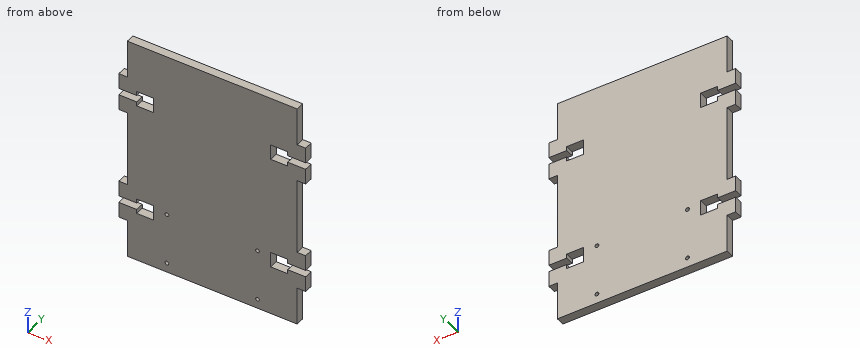
from build123d import *

# Parameters (mm, degrees)
SKETCH1_W           = 90
SKETCH1_H           = 20
SKETCH1_W_2         = 4.5
SKETCH1_H_2         = 8.2
SKETCH1_W_3         = 62
SKETCH1_H_3         = 3.6
SKETCH1_H_4         = 40
BOSS_EXTRUDE1_DEPTH = 4.5
CUT_EXTRUDE1_DEPTH  = 10


with BuildPart() as part:
    # Sketch1 → Boss-Extrude1 (new body)
    with BuildSketch(Plane(origin=(0, 0, 0), x_dir=(1, 0, 0), z_dir=(0, 1, 0))):
        with Locations((0, 50)):
            Rectangle(SKETCH1_W, SKETCH1_H)
        Polygon((-45, 40), (-45, 31.8), (-40, 31.8), (-40, 34), (-31, 34), (-31, 31.8), (31, 31.8), (31, 34), (40, 34), (40, 31.8), (45, 31.8), (45, 40), align=None)
        with Locations((-47.25, 35.9)):
            Rectangle(SKETCH1_W_2, SKETCH1_H_2)
        with Locations((-47.25, 24.1)):
            Rectangle(SKETCH1_W_2, SKETCH1_H_2)
        Polygon((-45, 28.2), (-45, 20), (45, 20), (45, 28.2), (40, 28.2), (40, 26), (31, 26), (31, 28.2), (-31, 28.2), (-31, 26), (-40, 26), (-40, 28.2), align=None)
        with Locations((0, 30)):
            Rectangle(SKETCH1_W_3, SKETCH1_H_3)
        Rectangle(SKETCH1_W, SKETCH1_H_4)
        Polygon((-45, -20), (-45, -28.2), (-40, -28.2), (-40, -26), (-31, -26), (-31, -28.2), (31, -28.2), (31, -26), (40, -26), (40, -28.2), (45, -28.2), (45, -20), align=None)
        with Locations((-47.25, -24.1)):
            Rectangle(SKETCH1_W_2, SKETCH1_H_2)
        with Locations((-47.25, -35.9)):
            Rectangle(SKETCH1_W_2, SKETCH1_H_2)
        Polygon((-45, -31.8), (-45, -40), (45, -40), (45, -31.8), (40, -31.8), (40, -34), (31, -34), (31, -31.8), (-31, -31.8), (-31, -34), (-40, -34), (-40, -31.8), align=None)
        with Locations((0, -30)):
            Rectangle(SKETCH1_W_3, SKETCH1_H_3)
        with Locations((47.25, -24.1)):
            Rectangle(SKETCH1_W_2, SKETCH1_H_2)
        with Locations((47.25, -35.9)):
            Rectangle(SKETCH1_W_2, SKETCH1_H_2)
        with Locations((47.25, 24.1)):
            Rectangle(SKETCH1_W_2, SKETCH1_H_2)
        with Locations((47.25, 35.9)):
            Rectangle(SKETCH1_W_2, SKETCH1_H_2)
        with Locations((0, -50)):
            Rectangle(SKETCH1_W, SKETCH1_H)
    extrude(amount=BOSS_EXTRUDE1_DEPTH)

    # Sketch2 → Cut-Extrude1 (cut)
    with BuildSketch(Plane(origin=(0, 4.5, 0), x_dir=(1, 0, 0), z_dir=(0, 1, 0))):
        with BuildLine():
            ThreePointArc((-23, 55), (-24.707106781, 55.707106781), (-24, 54))
            Line((-24, 54), (-24, 55))
            Line((-24, 55), (-23, 55))
        make_face()
        with BuildLine():
            Line((-24, 55), (-24, 54))
            ThreePointArc((-24, 54), (-23.292893219, 54.292893219), (-23, 55))
            Line((-23, 55), (-24, 55))
        make_face()
        with BuildLine():
            ThreePointArc((23, 55), (23.292893219, 54.292893219), (24, 54))
            Line((24, 54), (24, 55))
            Line((24, 55), (23, 55))
        make_face()
        with BuildLine():
            Line((24, 55), (24, 54))
            ThreePointArc((24, 54), (24.707106781, 54.292893219), (25, 55))
            ThreePointArc((25, 55), (24, 56), (23, 55))
            Line((23, 55), (24, 55))
        make_face()
        with BuildLine():
            ThreePointArc((24, 29), (23.292893219, 28.707106781), (23, 28))
            Line((23, 28), (24, 28))
            Line((24, 28), (24, 29))
        make_face()
        with BuildLine():
            Line((24, 28), (23, 28))
            ThreePointArc((23, 28), (24, 27), (25, 28))
            ThreePointArc((25, 28), (24.707106781, 28.707106781), (24, 29))
            Line((24, 29), (24, 28))
        make_face()
        with BuildLine():
            Line((-24, 29), (-24, 28))
            Line((-24, 28), (-23, 28))
            ThreePointArc((-23, 28), (-23.292893219, 28.707106781), (-24, 29))
        make_face()
        with BuildLine():
            Line((-23, 28), (-24, 28))
            Line((-24, 28), (-24, 29))
            ThreePointArc((-24, 29), (-24.707106781, 27.292893219), (-23, 28))
        make_face()
    extrude(amount=-CUT_EXTRUDE1_DEPTH, mode=Mode.SUBTRACT)


solid = part.part
Could you check a few things on this model? Use its own coordinates, in mm. Round coordinates to 2 decimals unless told otherwise and drop trailing zeros. Loops run counter-clockwise (first coordinate to the right, second up) from the corner with the lowest first, then second, coordinate; pieces in that order, holes last. Notation, with made-up numbers: (-32.5, -39) - (-10.5, -39) arc R18 ccw to (-10.5, -18) - close; hole circle Ø1 at (51, 6.25). An arc over 180 degrees is marked (long way). Write item = value, one per line.
1) I'm going to push flat-ended pins straight in: P1, Ø1.3, axis at x = -46.5, y = 3.5, coming from the -Z side; P2, Ø2, axis at y = 2, z = 2.5, coming from the -X side; P3, Ø1.3, axis at y = 3, z = -2.5, coming from the +X side. Where does each tip first touch, or does it pass through?
Computed:
P1 = -40
P2 = -45
P3 = 45
2) I need wall thicknesses on line 1 along X through (y, z) = (0.9, 32); line 2 along X through (y, z) = (2.75, -55); line 3 along Z through (x, y) = (33.5, 1.55). Which ranges of each line are inside material? Lowest first, please. Write a range as from..to.
Computed:
line_1 = -49.5..-40, -31..31, 40..49.5
line_2 = -45..-25, -23..23, 25..45
line_3 = -60..-34, -26..26, 34..60
3) Imagine slicing it at B-B (z = -1). Please give me the cut outline in (x, y), and give its area (3 significant figures).
Computed:
outline = (-45, 0) - (45, 0) - (45, 4.5) - (-45, 4.5) - close
area = 405 mm2
4) Imagine slicing it at A-A (y = 1.1). Give the number of separate pieces and of enclosed holes in the cut face, and give its area (3 significant figures).
Computed:
separate_pieces = 1
enclosed_holes = 4
area = 10,700 mm2
